Here's how the part is built. I have some questions about the finished solid (model axes, mm). Face numbers are marked on the shaded views. A direction names the side the tool comes from. Coordinates: 2 decimals unless noted, no trailing zeros. Write each loop counter-clockwise with the first axis right and the second up, starting at its lowest first coordinate (ties: lowest second). Pieces come first, ordered by that corner, then holes. Notation, with made-up numbers: M 64.5,0 L 108.5,0 A34 ccw 108.5,38 Z; hole C 72,49.5 d7. An arc over 180 degrees is marked long. Use a Markdown table: item, result.
```python
from build123d import *

# Parameters (mm, degrees)
SKETCH1_R               = 5
BOSS_EXTRUDE1_DEPTH     = 40
SKETCH2_R               = 6.5
BOSS_EXTRUDE2_DEPTH     = 8
CUT_EXTRUDE1_DEPTH      = 53.671192562
CUT_EXTRUDE1_DEPTH_BACK = 53.671192562
SKETCH3_R               = 5
SKETCH4_R               = 5
CUT_EXTRUDE2_DEPTH      = 61.052098431


with BuildPart() as part:
    # Sketch1 → Boss-Extrude1 (new body)
    with BuildSketch(Plane.XY):
        with BuildLine():
            ThreePointArc((-3.700263623, 14.536438667), (-4.104944851, 14.427384648), (-4.506421309, 14.30706703))
            ThreePointArc((-4.506421309, 14.30706703), (-5.549993278, 14.326184075), (-6.308323199, 13.609006518))
            ThreePointArc((-6.308323199, 13.609006518), (-6.686075337, 13.42744937), (-7.05860759, 13.235409283))
            ThreePointArc((-7.05860759, 13.235409283), (-8.087923512, 13.062444978), (-8.701560395, 12.218135975))
            ThreePointArc((-8.701560395, 12.218135975), (-9.039519546, 11.970258409), (-9.370421456, 11.713035547))
            ThreePointArc((-9.370421456, 11.713035547), (-10.350429211, 11.353879984), (-10.798476387, 10.411191465))
            ThreePointArc((-10.798476387, 10.411191465), (-11.085133758, 10.105434655), (-11.363136858, 9.791788434))
            ThreePointArc((-11.363136858, 9.791788434), (-12.260463457, 9.258672225), (-12.527663218, 8.249706316))
            ThreePointArc((-12.527663218, 8.249706316), (-12.753257036, 7.896482443), (-12.968894263, 7.53709371))
            ThreePointArc((-12.968894263, 7.53709371), (-13.752982325, 6.848171487), (-13.830235503, 5.807287313))
            ThreePointArc((-13.830235503, 5.807287313), (-13.987083441, 5.418624993), (-14.133011528, 5.025732299))
            ThreePointArc((-14.133011528, 5.025732299), (-14.777159874, 4.204464483), (-14.661835705, 3.167108106))
            ThreePointArc((-14.661835705, 3.167108106), (-14.744596495, 2.756242767), (-14.815846036, 2.343225603))
            ThreePointArc((-14.815846036, 2.343225603), (-15.298118968, 1.417579484), (-14.994144677, 0.419076831))
            ThreePointArc((-14.994144677, 0.419076831), (-15, 0), (-14.994144677, -0.419076831))
            ThreePointArc((-14.994144677, -0.419076831), (-15.298118968, -1.417579484), (-14.815846036, -2.343225603))
            ThreePointArc((-14.815846036, -2.343225603), (-14.744596495, -2.756242767), (-14.661835705, -3.167108106))
            ThreePointArc((-14.661835705, -3.167108106), (-14.777159874, -4.204464483), (-14.133011528, -5.025732299))
            ThreePointArc((-14.133011528, -5.025732299), (-13.987083441, -5.418624993), (-13.830235503, -5.807287313))
            ThreePointArc((-13.830235503, -5.807287313), (-13.752982325, -6.848171487), (-12.968894263, -7.53709371))
            ThreePointArc((-12.968894263, -7.53709371), (-12.753257036, -7.896482443), (-12.527663218, -8.249706316))
            ThreePointArc((-12.527663218, -8.249706316), (-12.260463457, -9.258672225), (-11.363136858, -9.791788434))
            ThreePointArc((-11.363136858, -9.791788434), (-11.085133758, -10.105434655), (-10.798476387, -10.411191465))
            ThreePointArc((-10.798476387, -10.411191465), (-10.350429211, -11.353879984), (-9.370421456, -11.713035547))
            ThreePointArc((-9.370421456, -11.713035547), (-9.039519546, -11.970258409), (-8.701560395, -12.218135975))
            ThreePointArc((-8.701560395, -12.218135975), (-8.087923512, -13.062444978), (-7.05860759, -13.235409283))
            ThreePointArc((-7.05860759, -13.235409283), (-6.686075337, -13.42744937), (-6.308323199, -13.609006518))
            ThreePointArc((-6.308323199, -13.609006518), (-5.549993278, -14.326184075), (-4.506421309, -14.30706703))
            ThreePointArc((-4.506421309, -14.30706703), (-4.104944851, -14.427384648), (-3.700263623, -14.536438667))
            ThreePointArc((-3.700263623, -14.536438667), (-2.82306468, -15.102062156), (-1.800774254, -14.891514768))
            ThreePointArc((-1.800774254, -14.891514768), (-1.384025392, -14.936012644), (-0.966196008, -14.968849831))
            ThreePointArc((-0.966196008, -14.968849831), (0, -15.363657622), (0.966196008, -14.968849831))
            ThreePointArc((0.966196008, -14.968849831), (1.384025392, -14.936012644), (1.800774254, -14.891514768))
            ThreePointArc((1.800774254, -14.891514768), (2.82306468, -15.102062156), (3.700263623, -14.536438667))
            ThreePointArc((3.700263623, -14.536438667), (4.104944851, -14.427384648), (4.506421309, -14.30706703))
            ThreePointArc((4.506421309, -14.30706703), (5.549993278, -14.326184075), (6.308323199, -13.609006518))
            ThreePointArc((6.308323199, -13.609006518), (6.686075337, -13.42744937), (7.05860759, -13.235409283))
            ThreePointArc((7.05860759, -13.235409283), (8.087923512, -13.062444978), (8.701560395, -12.218135975))
            ThreePointArc((8.701560395, -12.218135975), (9.039519546, -11.970258409), (9.370421456, -11.713035547))
            ThreePointArc((9.370421456, -11.713035547), (10.350429211, -11.353879984), (10.798476387, -10.411191465))
            ThreePointArc((10.798476387, -10.411191465), (11.085133758, -10.105434655), (11.363136858, -9.791788434))
            ThreePointArc((11.363136858, -9.791788434), (12.260463457, -9.258672225), (12.527663218, -8.249706316))
            ThreePointArc((12.527663218, -8.249706316), (12.753257036, -7.896482443), (12.968894263, -7.53709371))
            ThreePointArc((12.968894263, -7.53709371), (13.752982325, -6.848171487), (13.830235503, -5.807287313))
            ThreePointArc((13.830235503, -5.807287313), (13.987083441, -5.418624993), (14.133011528, -5.025732299))
            ThreePointArc((14.133011528, -5.025732299), (14.777159874, -4.204464483), (14.661835705, -3.167108106))
            ThreePointArc((14.661835705, -3.167108106), (14.744596495, -2.756242767), (14.815846036, -2.343225603))
            ThreePointArc((14.815846036, -2.343225603), (15.298118968, -1.417579484), (14.994144677, -0.419076831))
            ThreePointArc((14.994144677, -0.419076831), (15, 0), (14.994144677, 0.419076831))
            ThreePointArc((14.994144677, 0.419076831), (15.298118968, 1.417579484), (14.815846036, 2.343225603))
            ThreePointArc((14.815846036, 2.343225603), (14.744596495, 2.756242767), (14.661835705, 3.167108106))
            ThreePointArc((14.661835705, 3.167108106), (14.777159874, 4.204464483), (14.133011528, 5.025732299))
            ThreePointArc((14.133011528, 5.025732299), (13.987083441, 5.418624993), (13.830235503, 5.807287313))
            ThreePointArc((13.830235503, 5.807287313), (13.752982325, 6.848171487), (12.968894263, 7.53709371))
            ThreePointArc((12.968894263, 7.53709371), (12.753257036, 7.896482443), (12.527663218, 8.249706316))
            ThreePointArc((12.527663218, 8.249706316), (12.260463457, 9.258672225), (11.363136858, 9.791788434))
            ThreePointArc((11.363136858, 9.791788434), (11.085133758, 10.105434655), (10.798476387, 10.411191465))
            ThreePointArc((10.798476387, 10.411191465), (10.350429211, 11.353879984), (9.370421456, 11.713035547))
            ThreePointArc((9.370421456, 11.713035547), (9.039519546, 11.970258409), (8.701560395, 12.218135975))
            ThreePointArc((8.701560395, 12.218135975), (8.087923512, 13.062444978), (7.05860759, 13.235409283))
            ThreePointArc((7.05860759, 13.235409283), (6.686075337, 13.42744937), (6.308323199, 13.609006518))
            ThreePointArc((6.308323199, 13.609006518), (5.549993278, 14.326184075), (4.506421309, 14.30706703))
            ThreePointArc((4.506421309, 14.30706703), (4.104944851, 14.427384648), (3.700263623, 14.536438667))
            ThreePointArc((3.700263623, 14.536438667), (2.82306468, 15.102062156), (1.800774254, 14.891514768))
            ThreePointArc((1.800774254, 14.891514768), (1.384025392, 14.936012644), (0.966196008, 14.968849831))
            ThreePointArc((0.966196008, 14.968849831), (0, 15.363657622), (-0.966196008, 14.968849831))
            ThreePointArc((-0.966196008, 14.968849831), (-1.384025392, 14.936012644), (-1.800774254, 14.891514768))
            ThreePointArc((-1.800774254, 14.891514768), (-2.82306468, 15.102062156), (-3.700263623, 14.536438667))
        make_face()
        Circle(SKETCH1_R, mode=Mode.SUBTRACT)
    extrude(amount=BOSS_EXTRUDE1_DEPTH)

    # Sketch2 → Boss-Extrude2 (add)
    with BuildSketch(Plane.XY.offset(40)):
        Circle(SKETCH2_R)
    boss_extrude2 = extrude(amount=BOSS_EXTRUDE2_DEPTH)

    # Sketch3 → Cut-Extrude1 (cut, two sides: drawn at the far end of the back side and taken through both)
    with BuildSketch(Plane.XY.offset(48).offset(-CUT_EXTRUDE1_DEPTH_BACK)):
        Circle(SKETCH3_R)
    extrude(amount=CUT_EXTRUDE1_DEPTH + CUT_EXTRUDE1_DEPTH_BACK, mode=Mode.SUBTRACT)

    # Mirror1: Boss-Extrude2 across plane
    add(boss_extrude2.mirror(Plane(origin=(0, 0, 20), x_dir=(1, 0, 0), z_dir=(0, 0, -1))))

    # Sketch4 → Cut-Extrude2 (cut, through all)
    with BuildSketch(Plane(origin=(0, 0, -8), x_dir=(-1, 0, 0), z_dir=(0, 0, -1))):
        Circle(SKETCH4_R)
    extrude(amount=-CUT_EXTRUDE2_DEPTH, mode=Mode.SUBTRACT)


solid = part.part
```
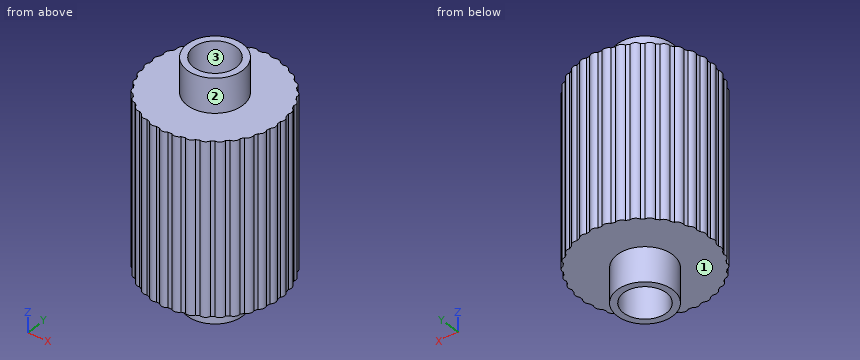
1. Suppose I cut it at A-A on x = 0. Write out the boundary of the cut face in (y, z), and give its area (3 significant figures).
Answers follow:
| item | result |
|---|---|
| outline | M -15.36,0 L -6.5,0 L -6.5,-8 L -5,-8 L -5,48 L -6.5,48 L -6.5,40 L -15.36,40 Z; M 5,-8 L 6.5,-8 L 6.5,0 L 15.36,0 L 15.36,40 L 6.5,40 L 6.5,48 L 5,48 Z |
| area | 877 mm2 |
2. Which directions (+Z, -Z, +X, -X, +Y, -Y) give clear straight access to the entire face, cutting with the end or side of a thin tool? Please do the marked faces 1, 2 and 3.
Answers follow:
| item | result |
|---|---|
| face 1 | -Z |
| face 2 | +Z |
| face 3 | +Z, -Z |
3. Will these pins go through, and if not, where does the flat tip stop? pin 1 Ø4 at (x, y) = (-7.5, -9) entering from -Z; pin 2 Ø15.5 at (x, y) = (0, -7) entering from +Z; pin 3 Ø12 at (y, z) = (12, 21) entering from +X; pin 4 Ø10 at (y, z) = (-11.5, 9) entering from -X.
Answers follow:
| item | result |
|---|---|
| pin 1 | stops at z = 0 |
| pin 2 | stops at z = 48 |
| pin 3 | stops at x = 13.9 |
| pin 4 | stops at x = -13.87 |
4. I need wall thicknesses on probe 1 along X at (y, z) = (0, 29); probe 2 along Y at (x, z) = (-2, 43); probe 3 along Z at (x, y) = (-9, -8). Which ranges of each line are inside material? Lowest first, please.
Answers follow:
| item | result |
|---|---|
| probe 1 | x = -15 to -5, 5 to 15 |
| probe 2 | y = -6.18 to -4.58, 4.58 to 6.18 |
| probe 3 | z = 0 to 40 |
5. Suppose I cut it at C-C on z = 43. Write out the boundary of the cut face in (x, y), and give its area (3 significant figures).
Answers follow:
| item | result |
|---|---|
| outline | C 0,0 d13; hole C 0,0 d10 |
| area | 54.2 mm2 |
6. Suppose I cut it at B-B on y = 4. Write out the boundary of the cut face in (x, z), and give its area (3 significant figures).
Answers follow:
| item | result |
|---|---|
| outline | M -14.82,0 L -5.12,0 L -5.12,-8 L -3,-8 L -3,48 L -5.12,48 L -5.12,40 L -14.82,40 Z; M 3,-8 L 5.12,-8 L 5.12,0 L 14.82,0 L 14.82,40 L 5.12,40 L 5.12,48 L 3,48 Z |
| area | 1,010 mm2 |
7. Suppose I cut it at D-D on y = 9. Write out the boundary of the cut face in (x, z).
Answers follow:
| item | result |
|---|---|
| outline | M -12.41,0 L 12.41,0 L 12.41,40 L -12.41,40 Z |
